Design review of the part built by this model. Coordinates are the model's own, in mm. Face numbers are marked on the shaded views. A direction names the side the tool comes from. Give positions to 0.01 mm unless a question says otherwise; leave off trailing zeros. Loops run counter-clockwise (first coordinate to the right, second up) from the corner with the lowest first, then second, coordinate; pieces in that order, holes last. Notation, with made-up numbers: M 57.5,2.25 L 61.5,2.25 A32 cw 61.5,39.25 Z; hole C 83,50 d3. An arc over 180 degrees is marked long. Use CSV: the item, a comma, the result in double quotes.
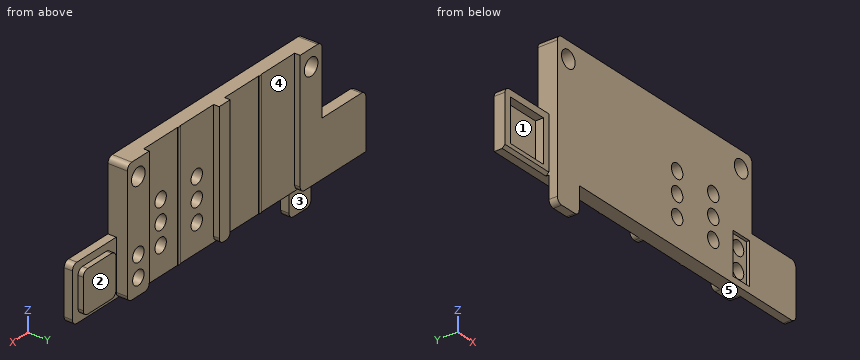
from build123d import *

# Parameters (mm, degrees)
SKETCH1_W             = 15.5
SKETCH1_H             = 45
BOSS_EXTRUDE1_DEPTH   = 5
BOSS_EXTRUDE1_2_DEPTH = 5
SKETCH1_R             = 2.6
BOSS_EXTRUDE1_3_DEPTH = 5
BOSS_EXTRUDE1_4_DEPTH = 5
SKETCH1_3_W           = 1
SKETCH1_3_H           = 45
BOSS_EXTRUDE2_DEPTH   = 5.2
SKETCH1_4_W           = 5
SKETCH1_4_H           = 45
SKETCH1_4_W_2         = 10
SKETCH1_4_R           = 2.6
BOSS_EXTRUDE3_DEPTH   = 7
SKETCH2_W             = 7.5
SKETCH2_H             = 15
CUT_EXTRUDE1_DEPTH    = 1.1
SKETCH3_R             = 3.1
CUT_EXTRUDE2_DEPTH    = 152.506600516
SKETCH5_W             = 20
SKETCH5_H             = 20
SKETCH5_W_2           = 14.9
SKETCH5_H_2           = 14.9
BOSS_EXTRUDE4_DEPTH   = 3
SKETCH5_3_W           = 14.9
SKETCH5_3_H           = 14.9
BOSS_EXTRUDE5_DEPTH   = 4.9
BOSS_EXTRUDE6_START   = 7
SKETCH5_4_W           = 20
SKETCH5_4_H           = 20
SKETCH5_4_W_2         = 15.2
SKETCH5_4_H_2         = 15.2
BOSS_EXTRUDE6_DEPTH   = 3.9
BOSS_EXTRUDE7_START   = 7
SKETCH5_5_W           = 15.2
SKETCH5_5_H           = 15.2
BOSS_EXTRUDE7_DEPTH   = 1
FILLET1_R             = 2
BOSS_EXTRUDE8_START   = -7
SKETCH6_W             = 10
SKETCH6_H             = 10
BOSS_EXTRUDE8_DEPTH   = 3
FILLET3_R             = 2
CHAMFER1_SIZE         = 1


with BuildPart() as part:
    # Sketch1 → Boss-Extrude1 (new body)
    with BuildSketch(Plane(origin=(0, 0, 0), x_dir=(1, 0, 0), z_dir=(0, 1, 0))):
        with Locations((73.25, 22.5)):
            Rectangle(SKETCH1_W, SKETCH1_H)
    extrude(amount=BOSS_EXTRUDE1_DEPTH)



with BuildPart() as body_2:
    # Sketch1 → Boss-Extrude1 2 (new body)
    with BuildSketch(Plane(origin=(0, 0, 0), x_dir=(1, 0, 0), z_dir=(0, 1, 0))):
        with Locations((89.75, 22.5)):
            Rectangle(SKETCH1_W, SKETCH1_H)
    extrude(amount=BOSS_EXTRUDE1_2_DEPTH)


with BuildPart() as body_3:
    # Sketch1 → Boss-Extrude1 3 (new body)
    with BuildSketch(Plane(origin=(0, 0, 0), x_dir=(1, 0, 0), z_dir=(0, 1, 0))):
        with Locations((110.25, 22.5)):
            Rectangle(SKETCH1_W, SKETCH1_H)
        with Locations(Location((110.25, 20, 0), (0, 0, 270))):
            Circle(SKETCH1_R, mode=Mode.SUBTRACT)
        with Locations(Location((110.25, 27.5, 0), (0, 0, 270))):
            Circle(SKETCH1_R, mode=Mode.SUBTRACT)
        with Locations(Location((110.25, 35, 0), (0, 0, 270))):
            Circle(SKETCH1_R, mode=Mode.SUBTRACT)
    extrude(amount=BOSS_EXTRUDE1_3_DEPTH)


with BuildPart() as body_4:
    # Sketch1 → Boss-Extrude1 4 (new body)
    with BuildSketch(Plane(origin=(0, 0, 0), x_dir=(1, 0, 0), z_dir=(0, 1, 0))):
        with Locations((126.75, 22.5)):
            Rectangle(SKETCH1_W, SKETCH1_H)
        with Locations(Location((126.75, 20, 0), (0, 0, 270))):
            Circle(SKETCH1_R, mode=Mode.SUBTRACT)
        with Locations(Location((126.75, 27.5, 0), (0, 0, 270))):
            Circle(SKETCH1_R, mode=Mode.SUBTRACT)
        with Locations(Location((126.75, 35, 0), (0, 0, 270))):
            Circle(SKETCH1_R, mode=Mode.SUBTRACT)
    extrude(amount=BOSS_EXTRUDE1_4_DEPTH)


with BuildPart() as part_1:
    add(part.part)

    add(body_2.part)  # Boss-Extrude2 merges body 2

    add(body_3.part)  # Boss-Extrude2 merges body 3

    add(body_4.part)  # Boss-Extrude2 merges body 4
    # Sketch1<3> → Boss-Extrude2 (add)
    with BuildSketch(Plane(origin=(0, 0, 0), x_dir=(1, 0, 0), z_dir=(0, 1, 0))):
        with Locations((81.5, 22.5)):
            Rectangle(SKETCH1_3_W, SKETCH1_3_H)
        with Locations((118.5, 22.5)):
            Rectangle(SKETCH1_3_W, SKETCH1_3_H)
    extrude(amount=BOSS_EXTRUDE2_DEPTH)

    # Sketch1<4> → Boss-Extrude3 (add)
    # profile 1 of 3: a face of its own
    with BuildSketch(Plane(origin=(0, 0, 0), x_dir=(1, 0, 0), z_dir=(0, 1, 0))):
        with Locations((100, 22.5)):
            Rectangle(SKETCH1_4_W, SKETCH1_4_H)
    # profile 2 of 3: a face of its own
    with BuildSketch(Plane(origin=(0, 0, 0), x_dir=(1, 0, 0), z_dir=(0, 1, 0))):
        with Locations((139.5, 22.5)):
            Rectangle(SKETCH1_4_W_2, SKETCH1_4_H)
        with Locations(Location((139.5, 31.5, 0), (0, 0, 270))):
            Circle(SKETCH1_4_R, mode=Mode.SUBTRACT)
        with Locations(Location((139.5, 39, 0), (0, 0, 270))):
            Circle(SKETCH1_4_R, mode=Mode.SUBTRACT)
    # profile 3 of 3: a face of its own
    with BuildSketch(Plane(origin=(0, 0, 0), x_dir=(1, 0, 0), z_dir=(0, 1, 0))):
        with Locations((60.5, 22.5)):
            Rectangle(SKETCH1_4_W_2, SKETCH1_4_H)
    extrude(amount=BOSS_EXTRUDE3_DEPTH)

    # Sketch2 → Cut-Extrude1 (cut)
    with BuildSketch(Plane(origin=(0, 0, 0), x_dir=(-1, 0, 0), z_dir=(0, -1, 0))):
        with Locations((-139.5, 35.25)):
            Rectangle(SKETCH2_W, SKETCH2_H)
    extrude(amount=-CUT_EXTRUDE1_DEPTH, mode=Mode.SUBTRACT)

    # Sketch3 → Cut-Extrude2 (cut, through all)
    with BuildSketch(Plane(origin=(0, 7, 0), x_dir=(1, 0, 0), z_dir=(0, 1, 0))):
        with Locations(Location((60.5, 6, 0), (0, 0, 270))):
            Circle(SKETCH3_R)
        with Locations(Location((139.5, 6, 0), (0, 0, 90))):
            Circle(SKETCH3_R)
    extrude(amount=-CUT_EXTRUDE2_DEPTH, mode=Mode.SUBTRACT)

    # Sketch5 → Boss-Extrude4 (add)
    # profile 1 of 2: a face of its own
    with BuildSketch(Plane(origin=(0, 0, 0), x_dir=(1, 0, 0), z_dir=(0, 1, 0))):
        with Locations((154.5, 35)):
            Rectangle(SKETCH5_W, SKETCH5_H)
        with Locations((154.5, 35)):
            Rectangle(SKETCH5_W_2, SKETCH5_H_2, mode=Mode.SUBTRACT)
    # profile 2 of 2: a face of its own
    with BuildSketch(Plane(origin=(0, 0, 0), x_dir=(1, 0, 0), z_dir=(0, 1, 0))):
        with Locations((154.5, 35)):
            Rectangle(SKETCH5_W_2, SKETCH5_H_2)
    extrude(amount=BOSS_EXTRUDE4_DEPTH)

    # Sketch5<3> → Boss-Extrude5 (add)
    with BuildSketch(Plane(origin=(0, 0, 0), x_dir=(1, 0, 0), z_dir=(0, 1, 0))):
        with Locations((154.5, 35)):
            Rectangle(SKETCH5_3_W, SKETCH5_3_H)
    extrude(amount=BOSS_EXTRUDE5_DEPTH)

    # Sketch5<4> → Boss-Extrude6 (add)
    with BuildSketch(Plane(origin=(0, 0, 0), x_dir=(1, 0, 0), z_dir=(0, 1, 0)).offset(BOSS_EXTRUDE6_START)):
        with Locations((45.5, 35)):
            Rectangle(SKETCH5_4_W, SKETCH5_4_H)
        with Locations((45.5, 35)):
            Rectangle(SKETCH5_4_W_2, SKETCH5_4_H_2, mode=Mode.SUBTRACT)
    extrude(amount=-BOSS_EXTRUDE6_DEPTH)

    # Sketch5<5> → Boss-Extrude7 (add)
    with BuildSketch(Plane(origin=(0, 0, 0), x_dir=(1, 0, 0), z_dir=(0, 1, 0)).offset(BOSS_EXTRUDE7_START)):
        with Locations((45.5, 35)):
            Rectangle(SKETCH5_5_W, SKETCH5_5_H)
    extrude(amount=-BOSS_EXTRUDE7_DEPTH)

    # Fillet1
    fillet1_edges = [part_1.edges().sort_by_distance(p)[0] for p in [
        (161.95, 3.95, -42.45),
        (147.05, 3.95, -42.45),
        (147.05, 3.95, -27.55),
        (161.95, 3.95, -27.55),
    ]]
    fillet(fillet1_edges, radius=FILLET1_R)

    # Sketch6 → Boss-Extrude8 (add)
    with BuildSketch(Plane(origin=(0, 7, 0), x_dir=(1, 0, 0), z_dir=(0, 1, 0)).offset(BOSS_EXTRUDE8_START)):
        with Locations((60.5, 50)):
            Rectangle(SKETCH6_W, SKETCH6_H)
    extrude(amount=BOSS_EXTRUDE8_DEPTH)

    # Fillet3
    fillet3_edges = [part_1.edges().sort_by_distance(p)[0] for p in [
        (164.5, 1.5, -45),
        (164.5, 1.5, -25),
        (35.5, 5.05, -25),
        (65.5, 1.5, -55),
        (55.5, 1.5, -55),
        (97.5, 6, -45),
        (102.5, 6, -45),
        (134.5, 6, -45),
        (144.5, 3.5, 0),
        (144.5, 5, -45),
        (55.5, 3.5, 0),
        (65.5, 6, -45),
    ]]
    fillet(fillet3_edges, radius=FILLET3_R)

    # Chamfer1
    chamfer1_edges = [part_1.edges().sort_by_distance(p)[0] for p in [
        (45.5, 3.1, -45),
    ]]
    chamfer(chamfer1_edges, length=CHAMFER1_SIZE)


solid = part_1.part
(1) We need section D-D on z = -20. State the section outline as (x, y) points.
A:
outline,"M 55.5,0 L 107.65,0 L 107.65,5 L 102.5,5 L 102.5,7 L 97.5,7 L 97.5,5 L 82,5 L 82,5.2 L 81,5.2 L 81,5 L 65.5,5 L 65.5,7 L 55.5,7 Z; M 112.85,0 L 124.15,0 L 124.15,5 L 119,5 L 119,5.2 L 118,5.2 L 118,5 L 112.85,5 Z; M 129.35,0 L 144.5,0 L 144.5,7 L 134.5,7 L 134.5,5 L 129.35,5 Z"
(2) Wall thickness on line 1 along X through (y, z) = (2.1, -27.5); line 2 along X through (y, z) = (5.5, -28.5); line 3 along X through (y, z) = (2, -20): over which ranges is each line inside the solid? List them lowest first. Write a range as [from, to].
A:
line 1,"[55.5, 107.65], [112.85, 124.15], [129.35, 164.5]"
line 2,"[35.5, 37.9], [53.1, 65.5], [97.5, 102.5], [134.5, 144.5]"
line 3,"[55.5, 107.65], [112.85, 124.15], [129.35, 144.5]"
(3) We need section A-A on z = -6. State the section outline as (x, y) points, then the cut area to 3 significant figures.
A:
outline,"M 55.5,0 L 57.4,0 L 57.4,7 L 55.5,7 Z; M 63.6,0 L 136.4,0 L 136.4,7 L 134.5,7 L 134.5,5 L 119,5 L 119,5.2 L 118,5.2 L 118,5 L 102.5,5 L 102.5,7 L 97.5,7 L 97.5,5 L 82,5 L 82,5.2 L 81,5.2 L 81,5 L 65.5,5 L 65.5,7 L 63.6,7 Z; M 142.6,0 L 144.5,0 L 144.5,7 L 142.6,7 Z"
area,"409 mm²"
(4) Machinability: for the marked faces 1, 2 and 3, which of the approach directions +Z, -Z, +X, -X, +Y, -Y give a long, thin tool a straight path to every point of the face, cutting with its end or side? Answer none if there is none.
A:
face 1,"-Y"
face 2,"+Z, -Z, +X, +Y"
face 3,"-Z, +X, -X, +Y"
(5) We need section C-C on x = 46.5. State the section outline as (y, z) points, then the cut area to 3 significant figures.
A:
outline,"M 3.1,-44 L 4.1,-45 L 7,-45 L 7,-25 L 3.1,-25 L 3.1,-27.4 L 6,-27.4 L 6,-42.6 L 3.1,-42.6 Z"
area,"33.4 mm²"
(6) Clearance check with flat-ended pins moving along their axes: P1, Ø9.5, axis at x = 45.5, z = -34, coming from the -Y side; P2, Ø0.8, axis at x = 81.5, z = -22, coming from the +Y side; P3, Ø5, axis at x = 62.5, z = -52, coming from the +Y side; P4, Ø7, axis at x = 139.5, z = -31.5, coming from the +Y side. State where each tip first meets the part, or that it passes through.
A:
P1,"y = 6"
P2,"y = 5.2"
P3,"y = 3"
P4,"y = 7"
(7) We need section B-B on x = 139.5. State the section outline as (y, z) points.
A:
outline,"M 0,-45 L 7,-45 L 7,-41.6 L 1.1,-41.6 L 1.1,-42.75 L 0,-42.75 Z; M 0,-27.75 L 1.1,-27.75 L 1.1,-28.9 L 7,-28.9 L 7,-9.1 L 0,-9.1 Z; M 0,-2.9 L 7,-2.9 L 7,0 L 0,0 Z; M 1.1,-36.4 L 7,-36.4 L 7,-34.1 L 1.1,-34.1 Z"
(8) The part is to be moulded in two halves that separate along X. For the marked faces 4 and 5, say which applies: released by +X, released by -X, zero draft, split by the parting line, or undercut.
A:
face 4,"undercut"
face 5,"zero draft"
